```python
from build123d import *

# Parameters (mm, degrees)
SKETCH_2_R               = 22.5
EXTRUDE_1_DEPTH          = 94
CUT_EXTRUDE_1_DEPTH      = 53
CUT_EXTRUDE_1_DEPTH_BACK = 53
SKETCH_3_W               = 19.263131719
SKETCH_3_H               = 15
EXTRUDE_3_DEPTH          = 16
EXTRUDE_3_DEPTH_BACK     = 19


with BuildPart() as part:
    # 草图2 → 凸台-拉伸1 (new body)
    with BuildSketch(Plane(origin=(0, 0, 0), x_dir=(0, 0, -1), z_dir=(1, 0, 0))):
        Circle(SKETCH_2_R)
    extrude(amount=EXTRUDE_1_DEPTH)

    # 草图3 → 切除-拉伸1 (cut, two sides: drawn at the far end of the back side and taken through both)
    with BuildSketch(Plane.XY.offset(-CUT_EXTRUDE_1_DEPTH_BACK)):
        with Locations((84.36843414, 7.5)):
            Rectangle(SKETCH_3_W, SKETCH_3_H)
        with Locations((84.36843414, -7.5)):
            Rectangle(SKETCH_3_W, SKETCH_3_H)
    extrude(amount=CUT_EXTRUDE_1_DEPTH + CUT_EXTRUDE_1_DEPTH_BACK, mode=Mode.SUBTRACT)

    # 草图4 → 凸台-拉伸3 (add, two sides: drawn at the far end of the back side and taken through both)
    with BuildSketch(Plane(origin=(0, 0, 0), x_dir=(1, 0, 0), z_dir=(0, 1, 0)).offset(-EXTRUDE_3_DEPTH_BACK)):
        with BuildLine():
            ThreePointArc((92.224417763, 0), (86.224417763, 6), (80.224417763, 0))
            Line((80.224417763, 0), (92.224417763, 0))
        make_face()
        with BuildLine():
            Line((92.224417763, 0), (80.224417763, 0))
            ThreePointArc((80.224417763, 0), (86.224417763, -6), (92.224417763, 0))
        make_face()
    extrude(amount=EXTRUDE_3_DEPTH + EXTRUDE_3_DEPTH_BACK)


solid = part.part
```
Geometry check sheet. Reference: the model listing, model coordinates, mm. A direction names the side the tool comes from. Coordinates: 2 decimals unless noted, no trailing zeros. Write each loop counter-clockwise with the first axis right and the second up, starting at its lowest first coordinate (ties: lowest second). Pieces come first, ordered by that corner, then holes. Notation, with made-up numbers: M -25.5,-9 L 0.5,-9 A15 cw 0.5,-2 Z; hole C -34,19 d11. An arc over 180 degrees is marked long. One line per item, written item: value. Start each with the question number.
(1) Sectioned sample at C-C, the plane x = 83. Enter the section's corners in (y, z), and give its area (3 significant figures).
(2) Release check for a two-part mould opening along Y. For faces 3 (the face through (74.737, 0, 0)), 4 (the face through (0, 0, 0)), 5 (the face through (46.34, 22.31, 2.93)) record: released by +Y, released by -Y, zero draft, split by the parting line, or undercut.
(3) Sectioned sample at D-D, the plane z = 10.5. Enter the section's corners in (x, y), and give its area (3 significant figures).
(4) Sectioned sample at B-B, the plane z = 0. Enter the section's corners in (x, y), and give its area (3 significant figures).
(5) Scan lines: line 1 along Y through (x, z) = (87.5, 16.5); line 2 along X through (y, z) = (6, 20); line 3 along Y through (x, z) = (80, 8). Record each from-to range of solid material in increasing order. Write a range as [from, to].
(6) Sectioned sample at A-A, the plane y = 0. Enter the section's corners in (x, z).
(7) Depth check by flat-ended pin: pin 1 (6 mm diameter, centred on x = 79.5, z = 8, fed in from +Y); pin 2 (3 mm diameter, centred on y = -8, z = 9, fed in from +X); pin 3 (1.5 mm diameter, centred on x = 26, y = -9, fed in from +Z); pin 4 (1.5 mm diameter, centred on x = 78, y = -9.5, fed in from +Z). Enter the tip coordinate at first touch or a pass-through.
(8) Tool access check on faces 1 (the face through (80, 15, 0)), 2 (the face through (94, 18, 0)). Record the directions out of +Z, -Z, +X, -X, +Y, -Y that give a thin tool (end or side, any length) a straight path to the whole face; none if there is none.
Filled sheet:
1. outline: M -15,-16.77 L -15,-5.06 L 15,-5.06 L 15,-16.77 A22.5 ccw 15,16.77 L 15,5.06 L -15,5.06 L -15,16.77 A22.5 ccw Z
1. area: 652 mm²
2. face 3: undercut
2. face 4: zero draft
2. face 5: split by the parting line
3. outline: M 0,-19.9 L 94,-19.9 L 94,-15 L 74.74,-15 L 74.74,15 L 94,15 L 94,19.9 L 0,19.9 Z
3. area: 3,160 mm²
4. outline: M 0,-22.5 L 94,-22.5 L 94,-15 L 92.22,-15 L 92.22,15 L 94,15 L 94,22.5 L 0,22.5 Z; hole M 74.74,-15 L 80.22,-15 L 80.22,15 L 74.74,15 Z
4. area: 4,010 mm²
5. line 1: [-15.3, -15], [15, 15.3]
5. line 2: [0, 74.74]
5. line 3: [-21.03, -15], [15, 21.03]
6. outline: M 0,-22.5 L 74.74,-22.5 L 74.74,22.5 L 0,22.5 Z; C 86.22,0 d12
7. pin 1: y = 21.94
7. pin 2: x = 74.74
7. pin 3: z = 20.93
7. pin 4: through
8. face 1: none
8. face 2: +Z, -Z, +X, +Y, -Y
